```python
from build123d import *

# Parameters (mm, degrees)
SKETCH_1_W          = 85
SKETCH_1_H          = 56
EXTRUDE_1_DEPTH     = 1
FILLET_1_R          = 3
SKETCH_2_R          = 1.375
CUT_EXTRUDE_1_DEPTH = 51.904322017
SKETCH_3_W          = 12
SKETCH_3_H          = 12
EXTRUDE_2_DEPTH     = 1.2
SKETCH_4_W          = 8.2
SKETCH_4_H          = 8.2
EXTRUDE_3_DEPTH     = 1


with BuildPart() as part:
    # Эскиз1 → Бобышка-Вытянуть1 (new body)
    with BuildSketch(Plane(origin=(0, 0, 0), x_dir=(1, 0, 0), z_dir=(0, 1, 0))):
        Rectangle(SKETCH_1_W, SKETCH_1_H)
    extrude(amount=EXTRUDE_1_DEPTH)

    # Скругление1
    fillet_1_edges = [part.edges().sort_by_distance(p)[0] for p in [
        (-42.5, 0.5, -28),
        (42.5, 0.5, -28),
        (42.5, 0.5, 28),
        (-42.5, 0.5, 28),
    ]]
    fillet(fillet_1_edges, radius=FILLET_1_R)

    # Эскиз2 → Вырез-Вытянуть1 (cut, through all)
    with BuildSketch(Plane(origin=(0, 1, 0), x_dir=(1, 0, 0), z_dir=(0, 1, 0))):
        with Locations(Location((19, 24.5, 0), (0, 0, 270))):
            Circle(SKETCH_2_R)
        with Locations(Location((-39, 24.5, 0), (0, 0, 270))):
            Circle(SKETCH_2_R)
        with Locations(Location((-39, -24.5, 0), (0, 0, 270))):
            Circle(SKETCH_2_R)
        with Locations(Location((19, -24.5, 0), (0, 0, 270))):
            Circle(SKETCH_2_R)
    extrude(amount=-CUT_EXTRUDE_1_DEPTH, mode=Mode.SUBTRACT)

    # Эскиз3 → Бобышка-Вытянуть2 (add)
    with BuildSketch(Plane(origin=(0, 1, 0), x_dir=(1, 0, 0), z_dir=(0, 1, 0))):
        with Locations((-13.3, 1.8)):
            Rectangle(SKETCH_3_W, SKETCH_3_H)
    extrude(amount=EXTRUDE_2_DEPTH)

    # Эскиз4 → Бобышка-Вытянуть3 (add)
    with BuildSketch(Plane(origin=(0, 1, 0), x_dir=(1, 0, 0), z_dir=(0, 1, 0))):
        with Locations((14.8, 5.8)):
            Rectangle(SKETCH_4_W, SKETCH_4_H)
    extrude(amount=EXTRUDE_3_DEPTH)


solid = part.part
```
Here's how the part is built. I have some questions about the finished solid (model axes, mm). A direction names the side the tool comes from. Round coordinates to 2 decimals unless told otherwise and drop trailing zeros. Loops run counter-clockwise (first coordinate to the right, second up) from the corner with the lowest first, then second, coordinate; pieces in that order, holes last.
1. For faces 1 (the face through (-41.64, 0.51, -27.1)), 2 (the face through (15, 2, -6)), which set-ups out of +Z, -Z, +X, -X, +Y, -Y let a thin tool reach every point of the face, with its end or its side?
Answers:
face 1: -Z, -X, +Y, -Y
face 2: +Z, -Z, +X, +Y
2. Suppose I cut it at A-A, the plane y = 1.5. Please give me the cut outline in (x, z), and give its area (3 significant figures).
Answers:
outline: (-19.3, -7.8) - (-7.3, -7.8) - (-7.3, 4.2) - (-19.3, 4.2) - close; (10.7, -9.9) - (18.9, -9.9) - (18.9, -1.7) - (10.7, -1.7) - close
area: 211 mm2
3. Thinking about a two-plate mould opening in Z: for faces 3 (the face through (-38.071, 0.507, 23.487)), 4 (the face through (-38.071, 0.507, -25.513)), 5 (the face through (41.64, 0.51, -27.1)), 6 (the face through (41.6, 0.51, 27.14)), which applies, released by +Z, released by -Z, zero draft, split by the parting line, or undercut?
Answers:
face 3: undercut
face 4: undercut
face 5: released by -Z
face 6: released by +Z
4. Suppose I cut it at B-B, the plane z = -21. Please give me the cut outline in (x, y), and give its area (3 significant figures).
Answers:
outline: (-42.5, 0) - (42.5, 0) - (42.5, 1) - (-42.5, 1) - close
area: 85.0 mm2
5. If I drill on probe 1 along X at (y, z) = (0.55, 24.5) (3 decimals); probe 2 along Y at (x, z) = (-29, -1); probe 3 along X at (y, z) = (1.8, -7), over which ranges is the centre line in solid material (lowest first)?
Answers:
probe 1: x = -42.5 to -40.375, -37.625 to 17.625, 20.375 to 42.5
probe 2: y = 0 to 1
probe 3: x = -19.3 to -7.3, 10.7 to 18.9
6. Suppose I cut it at C-C, the plane x = -28.5. Please give me the cut outline in (y, z), and give its area (3 significant figures).
Answers:
outline: (0, -28) - (1, -28) - (1, 28) - (0, 28) - close
area: 56.0 mm2
7. Will these pins go through, and if not, where does the flat tip stop? pin 1 (2.5 mm diameter, centred on x = 19, z = 24.5, fed in from +Y); pin 2 (2 mm diameter, centred on x = -31, z = -18, fed in from +Y); pin 3 (0.5 mm diameter, centred on x = 14.5, y = 1.5, fed in from -Z); pin 4 (1 mm diameter, centred on x = -16, y = 2, fed in from +Z).
Answers:
pin 1: passes through
pin 2: stops at y = 1
pin 3: stops at z = -9.9
pin 4: stops at z = 4.2
